Work out the finished part from the listing and answer in its coordinate system (mm). Face numbers are marked on the shaded views. A direction names the side the tool comes from. Coordinates: 2 decimals unless noted, no trailing zeros. Write each loop counter-clockwise with the first axis right and the second up, starting at its lowest first coordinate (ties: lowest second). Pieces come first, ordered by that corner, then holes. Notation, with made-up numbers: M 89,29.5 L 124,29.5 A17 ccw 124,48.5 Z; hole C 62,40.5 d11. An arc over 180 degrees is marked long. Answer as CSV lines item,"result". Start each with the question number.
(1) Flat-ended cylindrical pins translate along their axes: P1, Ø3, axis at y = 117.5, z = -2.5, coming from the +X side; P2, Ø4, axis at x = 31.47, y = 31.47, coming from the -Z side; P3, Ø4, axis at x = -31.47, y = 208.23, coming from the +Z side. Find the tip coordinate at first contact, or state that the pin passes through.
(2) A cutting plane is placed at C-C on x = 12. Give the vertices of the cut face in (y, z), then the cut area to 3 significant figures.
(3) A cutting plane is placed at D-D on y = 77. Give the vertices of the cut face in (x, z), then the cut area to 3 significant figures.
(4) A cutting plane is placed at A-A on z = -8. Give the vertices of the cut face in (x, y).
(5) For the marked faces 4, 5 and 6, determine the directions among +Z, -Z, +X, -X, +Y, -Y from which every point of the face is accessible in a straight line to the end or side of a thin tool.
(6) Find the intervals of material crossed by L1, parallel to X at y = 181, z = -7; L2, parallel to X at y = 151.5, z = -2; L3, parallel to Y at x = -8.5, z = -7.25, in increasing order. Write a range as [from, to].
(7) A cutting plane is placed at B-B on y = 131. Give the vertices of the cut face in (x, z).
(8) The mould has two halves that part along Y. Classify the marked faces 1, 2 and 3: released by +Y, released by -Y, zero draft, split by the parting line, or undercut.
from build123d import *

# Parameters (mm, degrees)
SKETCH1_R           = 48.25
BOSS_EXTRUDE1_DEPTH = 10
SKETCH2_W           = 17.162038191
SKETCH2_H           = 56.822210482
SKETCH2_W_2         = 16.152506533
SKETCH2_H_2         = 65.186901365
CUT_EXTRUDE1_DEPTH  = 8
SKETCH3_R           = 32
CUT_EXTRUDE2_DEPTH  = 10
SKETCH4_R           = 1.75
CUT_EXTRUDE3_DEPTH  = 10
SKETCH9_R           = 3
CUT_EXTRUDE4_DEPTH  = 3.5
SKETCH12_R          = 48.25
BOSS_EXTRUDE4_DEPTH = 10
SKETCH13_W          = 17.162038191
SKETCH13_H          = 240.265998925
SKETCH13_W_2        = 16.152506533
SKETCH13_H_2        = 226.18217938
CUT_EXTRUDE5_DEPTH  = 5
SKETCH14_R          = 30
CUT_EXTRUDE6_DEPTH  = 10
CUT_EXTRUDE7_DEPTH  = 10
CUT_EXTRUDE8_DEPTH  = 10
SKETCH19_R          = 1.75
CUT_EXTRUDE9_DEPTH  = 10
BOSS_EXTRUDE5_DEPTH = 10
SKETCH21_R          = 32
CUT_EXTRUDE11_DEPTH = 10
SKETCH23_R          = 3
CUT_EXTRUDE13_DEPTH = 3.5
CUT_EXTRUDE14_START = -5
SKETCH24_R          = 48.25
CUT_EXTRUDE14_DEPTH = 5


with BuildPart() as part:
    # Sketch1 → Boss-Extrude1 (new body)
    with BuildSketch(Plane.XY):
        Circle(SKETCH1_R)
    extrude(amount=-BOSS_EXTRUDE1_DEPTH)

    # Sketch2 → Cut-Extrude1 (cut)
    with BuildSketch(Plane.XY):
        with Locations((-54.831019095, 0)):
            Rectangle(SKETCH2_W, SKETCH2_H)
        with Locations((54.326253267, -4.182345442)):
            Rectangle(SKETCH2_W_2, SKETCH2_H_2)
    extrude(amount=-CUT_EXTRUDE1_DEPTH, mode=Mode.SUBTRACT)

    # Sketch3 → Cut-Extrude2 (cut)
    with BuildSketch(Plane.XY):
        Circle(SKETCH3_R)
    extrude(amount=-CUT_EXTRUDE2_DEPTH, mode=Mode.SUBTRACT)

    # Sketch4 → Cut-Extrude3 (cut)
    with BuildSketch(Plane.XY):
        with Locations((-42.5, 0)):
            Circle(SKETCH4_R)
        with Locations((0, -44.5)):
            Circle(SKETCH4_R)
        with Locations((0, 44.5)):
            Circle(SKETCH4_R)
        with Locations((42.5, 0)):
            Circle(SKETCH4_R)
        with Locations((-31.466251763, -31.466251763)):
            Circle(SKETCH4_R)
        with Locations((31.466251763, -31.466251763)):
            Circle(SKETCH4_R)
        with Locations((31.466251763, 31.466251763)):
            Circle(SKETCH4_R)
        with Locations((-31.466251763, 31.466251763)):
            Circle(SKETCH4_R)
    extrude(amount=-CUT_EXTRUDE3_DEPTH, mode=Mode.SUBTRACT)

    # Sketch9 → Cut-Extrude4 (cut)
    with BuildSketch(Plane.XY):
        with Locations((-42.5, 0)):
            Circle(SKETCH9_R)
        with Locations((42.5, 0)):
            Circle(SKETCH9_R)
        with Locations((31.466251763, 31.466251763)):
            Circle(SKETCH9_R)
        with Locations((-31.466251763, 31.466251763)):
            Circle(SKETCH9_R)
        with Locations((-31.466251763, -31.466251763)):
            Circle(SKETCH9_R)
        with Locations((31.466251763, -31.466251763)):
            Circle(SKETCH9_R)
        with Locations((0, -44.5)):
            Circle(SKETCH9_R)
        with Locations((0, 44.5)):
            Circle(SKETCH9_R)
    extrude(amount=-CUT_EXTRUDE4_DEPTH, mode=Mode.SUBTRACT)

    # Sketch17 → Cut-Extrude7 (cut)
    with BuildSketch(Plane.XY):
        Polygon((0, 0), (-69.304284442, 39.961433382), (-69.278270797, -65.322297693), (63.970930278, -62.407226987), (69.259758702, 40.038554227), align=None)
    extrude(amount=-CUT_EXTRUDE7_DEPTH, mode=Mode.SUBTRACT)



with BuildPart() as body_2:
    # Sketch12 → Boss-Extrude4 (new body)
    with BuildSketch(Plane.XY):
        with Locations((0, 239.694162197)):
            Circle(SKETCH12_R)
    extrude(amount=-BOSS_EXTRUDE4_DEPTH)

    # Sketch13 → Cut-Extrude5 (cut)
    with BuildSketch(Plane.XY):
        with Locations((-54.831019095, 316.834631882)):
            Rectangle(SKETCH13_W, SKETCH13_H)
        with Locations((54.326253267, 300.281083797)):
            Rectangle(SKETCH13_W_2, SKETCH13_H_2)
    extrude(amount=-CUT_EXTRUDE5_DEPTH, mode=Mode.SUBTRACT)

    # Sketch14 → Cut-Extrude6 (cut)
    with BuildSketch(Plane.XY):
        with Locations((0, 239.694162197)):
            Circle(SKETCH14_R)
    extrude(amount=-CUT_EXTRUDE6_DEPTH, mode=Mode.SUBTRACT)

    # Sketch18 → Cut-Extrude8 (cut)
    with BuildSketch(Plane.XY):
        Polygon((0, 239.694162197), (-69.284269814, 199.69803793), (-69.066382196, 357.511219566), (54.70167511, 362.333351669), (69.279794575, 199.690286588), align=None)
    extrude(amount=-CUT_EXTRUDE8_DEPTH, mode=Mode.SUBTRACT)

    # Sketch19 → Cut-Extrude9 (cut)
    with BuildSketch(Plane.XY):
        with Locations((0, 195.194162197)):
            Circle(SKETCH19_R)
        with Locations((-31.466251763, 208.227910434)):
            Circle(SKETCH19_R)
        with Locations((31.466251763, 208.227910434)):
            Circle(SKETCH19_R)
    extrude(amount=-CUT_EXTRUDE9_DEPTH, mode=Mode.SUBTRACT)


with BuildPart() as part_1:
    add(part.part)

    add(body_2.part)  # Boss-Extrude5 merges body 2
    # Sketch10 → Boss-Extrude5 (add)
    with BuildSketch(Plane.XY):
        with BuildLine():
            Line((-17.5, 179.53997423), (-17.5, 194.729592811))
            ThreePointArc((-17.5, 194.729592811), (-23.743486454, 197.690479608), (-29.5, 201.512851323))
            Line((-29.5, 201.512851323), (-29.5, 38.181310873))
            ThreePointArc((-29.5, 38.181310873), (-16.697131744, 45.268844601), (-2.358379682, 48.192328697))
            Line((-2.358379682, 48.192328697), (17.5, 59.53997423))
            Line((17.5, 59.53997423), (17.5, 44.964569385))
            ThreePointArc((17.5, 44.964569385), (23.743486454, 42.003682588), (29.5, 38.181310873))
            Line((29.5, 38.181310873), (29.5, 201.512851323))
            ThreePointArc((29.5, 201.512851323), (17.261915402, 194.637655711), (3.562842942, 191.575884483))
            Line((3.562842942, 191.575884483), (-17.5, 179.53997423))
        make_face()
        Polygon((17.5, 187.53997423), (17.5, 147.53997423), (-17.5, 167.53997423), align=None, mode=Mode.SUBTRACT)
        Polygon((17.5, 135.53997423), (-17.5, 115.53997423), (-17.5, 155.53997423), align=None, mode=Mode.SUBTRACT)
        Polygon((17.5, 123.53997423), (17.5, 83.53997423), (-17.5, 103.53997423), align=None, mode=Mode.SUBTRACT)
        Polygon((17.5, 71.53997423), (-17.5, 51.53997423), (-17.5, 91.53997423), align=None, mode=Mode.SUBTRACT)
    extrude(amount=-BOSS_EXTRUDE5_DEPTH)

    # Sketch21 → Cut-Extrude11 (cut)
    with BuildSketch(Plane.XY):
        with Locations((0, 239.694162197)):
            Circle(SKETCH21_R)
    extrude(amount=-CUT_EXTRUDE11_DEPTH, mode=Mode.SUBTRACT)

    # Sketch23 → Cut-Extrude13 (cut)
    with BuildSketch(Plane.XY):
        with Locations((-31.466251763, 208.227910434)):
            Circle(SKETCH23_R)
        with Locations((0, 195.194162197)):
            Circle(SKETCH23_R)
        with Locations((31.466251763, 208.227910434)):
            Circle(SKETCH23_R)
        with Locations((0, 44.5)):
            Circle(SKETCH23_R)
    extrude(amount=-CUT_EXTRUDE13_DEPTH, mode=Mode.SUBTRACT)

    # Sketch24 → Cut-Extrude14 (cut)
    with BuildSketch(Plane(origin=(0, 0, -10), x_dir=(-1, 0, 0), z_dir=(0, 0, -1)).offset(CUT_EXTRUDE14_START)):
        with Locations((0, 239.694162197)):
            Circle(SKETCH24_R)
        Circle(SKETCH24_R)
    extrude(amount=CUT_EXTRUDE14_DEPTH, mode=Mode.SUBTRACT)


solid = part_1.part
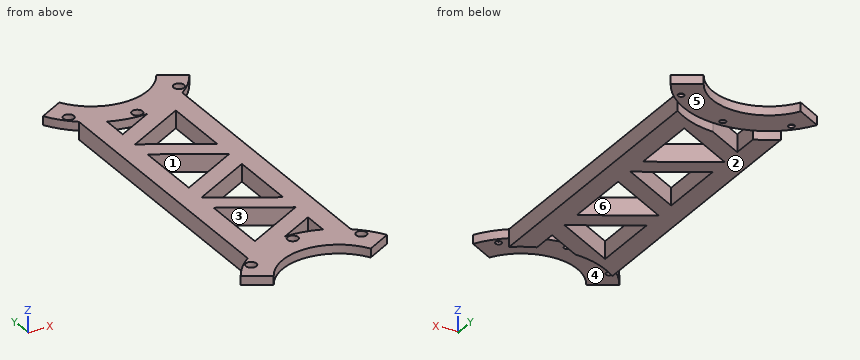
Here are the results:
1,P1,"stops at x = 29.5"
1,P2,"stops at z = -5"
1,P3,"stops at z = -3.5"
2,outline,"M 29.66,-5 L 46.73,-5 L 46.73,0 L 29.66,0 Z; M 56.4,-10 L 68.4,-10 L 68.4,0 L 56.4,0 Z; M 74.68,-10 L 86.68,-10 L 86.68,0 L 74.68,0 Z; M 120.4,-10 L 132.4,-10 L 132.4,0 L 120.4,0 Z; M 138.68,-10 L 150.68,-10 L 150.68,0 L 138.68,0 Z; M 184.4,-10 L 192.96,-10 L 192.96,-5 L 210.03,-5 L 210.03,0 L 184.4,0 Z"
2,area,"736 mm^2"
3,outline,"M -29.5,-10 L -17.5,-10 L -17.5,0 L -29.5,0 Z; M 7.94,-10 L 29.5,-10 L 29.5,0 L 7.94,0 Z"
3,area,"336 mm^2"
4,outline,"M -29.5,38.18 A48.25 cw -2.36,48.19 L 17.5,59.54 L 17.5,44.96 A48.25 cw 29.5,38.18 L 29.5,201.51 A48.25 cw 3.56,191.58 L -17.5,179.54 L -17.5,194.73 A48.25 cw -29.5,201.51 Z; hole M -17.5,51.54 L 17.5,71.54 L -17.5,91.54 Z; hole M -17.5,103.54 L 17.5,83.54 L 17.5,123.54 Z; hole M -17.5,115.54 L 17.5,135.54 L -17.5,155.54 Z; hole M -17.5,167.54 L 17.5,147.54 L 17.5,187.54 Z"
5,face 4,"-Z, -Y"
5,face 5,"-Z, +Y"
5,face 6,"+Z, -Z"
6,L1,"x = [-29.5, -17.5], [-14.94, 6.06], [17.5, 29.5]"
6,L2,"x = [-29.5, -17.5], [-10.43, 10.57], [17.5, 29.5]"
6,L3,"y = [47.5, 56.68], [86.4, 98.4], [108.68, 120.68], [150.4, 162.4], [172.68, 184.68]"
7,outline,"M -29.5,-10 L -17.5,-10 L -17.5,0 L -29.5,0 Z; M 9.56,-10 L 29.5,-10 L 29.5,0 L 9.56,0 Z"
8,face 1,"undercut"
8,face 2,"zero draft"
8,face 3,"undercut"
